from build123d import *

# Parameters (mm, degrees)
F0_W     = 42.9752953351
F0_H     = 26.1746868491
F1_DEPTH = 25.4
F2_R     = 5.0570652765
F3_DEPTH = 25.401


# Not quite as in the source:
# - the program builds the solid bodies; features that only make, move or delete a surface that nothing else refers to are left out


with BuildPart() as f1:
    # F0 (on Front) → F1 (new body)
    with BuildSketch(Plane.XZ):
        with Locations((21.4876476675, 13.0873434246)):
            Rectangle(F0_W, F0_H)
    extrude(amount=-F1_DEPTH)

    # F2 (on face) → F3 (cut, through all)
    with BuildSketch(Plane.XZ):
        with Locations((14.6032562479, 13.0873434246)):
            Circle(F2_R)
    extrude(amount=-F3_DEPTH, mode=Mode.SUBTRACT)


solid = f1.part
For this review, take the finished solid that the model builds, in its own axes (mm). Give positions to 0.01 mm unless a question says otherwise; leave off trailing zeros. Loops run counter-clockwise (first coordinate to the right, second up) from the corner with the lowest first, then second, coordinate; pieces in that order, holes last. Notation, with made-up numbers: M -29.75,78 L 15.25,78 A17 ccw 15.25,111 Z; hole C 44,4 d8. An arc over 180 degrees is marked long. Put each result on its own line as item: value. Start each with the question number.
(1) Add section C-C, the plane y = 9. Write out the cut boundary in (x, z), then the cut area to 3 significant figures.
(2) Add section A-A, the plane z = 14.25. Write out the cut boundary in (x, y), then the cut area to 3 significant figures.
(3) Wall thickness on L1, parallel to X at y = 24.25, z = 13.25; L2, parallel to Z at x = 10, y = 14.25; L3, parallel to X at y = 16.25, z = 17.75: over which ranges is each line inside the solid? List them lowest first.
(4) The part is to be moulded in two halves that separate along X. For faces 1 (the flat face through (0, 13, 13)), 2 (the cylindrical face through (19.275, 12.522, 11.15)), 3 (the flat face through (21, 13, 0)), 4 (the flat face through (42.975, 13, 13)), say which applies: +X half, -X half, draft (parallel to the pull), parting line (faces both ways), or undercut.
(5) Add section B-B, the plane x = 18. Write out the cut boundary in (y, z).
Result:
1. outline: M 0,0 L 42.98,0 L 42.98,26.17 L 0,26.17 Z; hole C 14.6,13.09 d10.11
1. area: 1,040 mm^2
2. outline: M 0,0 L 9.68,0 L 9.68,25.4 L 0,25.4 Z; M 19.52,0 L 42.98,0 L 42.98,25.4 L 19.52,25.4 Z
2. area: 842 mm^2
3. L1: x = 0 to 9.55, 19.66 to 42.98
3. L2: z = 0 to 10.99, 15.18 to 26.17
3. L3: x = 0 to 12.65, 16.56 to 42.98
4. face 1: -X half
4. face 2: undercut
4. face 3: draft
4. face 4: +X half
5. outline: M 0,0 L 25.4,0 L 25.4,9.34 L 0,9.34 Z; M 0,16.83 L 25.4,16.83 L 25.4,26.17 L 0,26.17 Z
